Autodesk Inventor part; units mm, degrees
ref_plane "YZ Plane" through (0, 0, 0) normal (1, 0, 0) x (0, 1, 0)
ref_plane "XZ Plane" through (0, 0, 0) normal (0, 1, 0) x (-1, 0, 0)
ref_plane "XY Plane" through (0, 0, 0) normal (0, 0, 1) x (1, 0, 0)
sketch "Sketch1" plane through (0, 0, 0) normal (0, 1, 0) x (-1, 0, 0)
  line L0 (0, 0) -> (0, 29.0928)
  line L1 (0, 29.0928) -> (-0.9185, 29.0928)
  line L2 (-0.9185, 29.0928) -> (-3.25, 24.0928)
  line L3 (-3.25, 24.0928) -> (-2.4, 24.0928)
  line L4 (-2.4, 24.0928) -> (-2.4, 20.2928)
  line L5 (-2.4, 20.2928) -> (-3, 20.2928)
  line L6 (-3, 20.2928) -> (-3, 6)
  line L7 (-3, 6) -> (-1.5, 6)
  line L8 (-1.5, 6) -> (-1.5, 0)
  line L9 (-1.5, 0) -> (0, 0)
  arc A0 (-6.8684, 22.0226) -> (0, 20.2928) centre (0, 34.7935) ccw
  arc A1 (-6.6316, 22.4629) -> (-2.4, 21) centre (0, 34.7935) ccw
  arc A2 (-6.6316, 22.4629) -> (-6.8684, 22.0226) centre (-6.75, 22.2428) ccw
  line L10 (-2.4, 21) -> (0, 21)
  point P0 (0, 10)
  dimension "d0" = 3
  dimension "d1" = 6
  dimension "d3" = 6
  dimension "d4" = 5
  dimension "d5" = 6.5
  dimension "d9" = 8.8
  dimension "d10" = 25
  dimension "d11" = 4.8
  dimension "d15" = 15
  dimension "d17" = 14
  dimension "d18" = 0.5
  dimension "d19" = 1.6
revolve "Revolution1" add sketch "Sketch1" angle 360 about axis through (0, 0, 0) along (0, 0, 1) contours L9 L8 L7 L6 L5 L4 A0 L0 | A0 L4 L10 L0 | L10 L4 L3 L2 L1 L0
extrude "Extrusion1" add sketch "Sketch1" along normal mid plane 5.5 contours A0 L4 L10 L0 | A0 A2 A1 L4
mirror "Mirror1" about plane through (0, 0, 20.2928) normal (-1, 0, 0) of "Extrusion1"
properties part number "WBN-315" material "Acetal Resin, White"
Source: CAD feature listing. Evaluate the final solid. Frame: model axes, mm. A direction names the side the tool comes from. Coordinates: 2 decimals unless noted, no trailing zeros. Order: outer loops, then holes, each group sorted by start corner. A loop starts at its lowest first (then second) coordinate and runs counter-clockwise, first axis right, second up. Notation, with made-up numbers: M 76.5,26 L 132.5,26 A31 cw 132.5,52 Z; hole C -34.5,46.25 d11. An arc over 180 degrees is marked long. Write each question's results on one line, items separated by ' | '. Start each with the question number.
Item 1: First-contact query: pin 1 Ø4 at (x, z) = (-4, 14) entering from -Y; pin 2 Ø1.5 at (x, z) = (3.5, 15.5) entering from +Y; pin 3 Ø8 at (x, z) = (5.5, 14.5) entering from -Y. Flat tips, straight axial feed; report the tip coordinate or a pass-through.
Item 2: Set-up query: faces 1 (the face through (1.3, -1.3, 6)), 2 (the face through (0, 2.75, 20.8)), 3 (the face through (0.01, 2.59, 21)), 4 (the face through (1.29, -2.024, 22.525)), 5 (the face through (4.54, -0.04, 21.55)). Return all of +Z, -Z, +X, -X, +Y, -Y with unobstructed straight access to the full face (end or side cutting, diameter ignored); none if empty.
Item 3: Cut plane A-A (z = 17). Return loops of the section in (x, y).
Item 4: Cut plane B-B (x = -3.75). Return loops of the section in (y, z).
Item 5: Draft query along X for faces 6 (the face through (-1.5, -0.07, 2.96)), 7 (the face through (-4.6, -0.04, 21.57)), 8 (the face through (0, -2.75, 20.8)). Return one class per face: pulls with the +X half, pulls with the -X half, needs draft (parallel to the pull), parting line crosses it, or undercut.
Item 6: Cut plane C-C (x = 6). Return loops of the section in (y, z).
Item 7: Line query: probe 1 along Z at (x, y) = (2.75, 0.5); probe 2 along X at (y, z) = (1.75, 22.25); probe 3 along X at (y, z) = (-0.5, 15.5). Output: solid intervals per line, ascending.
Checked values:
1) pin 1: stops at y = -2.24 | pin 2: stops at y = 1.2 | pin 3: stops at y = -2.6
2) face 1: -Z | face 2: +X, -X, +Y | face 3: +Y | face 4: none | face 5: +Y, -Y
3) outline: C 0,0 d6
4) outline: M -2.75,20.79 L 2.75,20.79 L 2.75,21.3 L -2.75,21.3 Z
5) face 6: parting line crosses it | face 7: undercut | face 8: needs draft
6) outline: M -2.75,21.59 L 2.75,21.59 L 2.75,22.14 L -2.75,22.14 Z
7) probe 1: z = 6 to 20.29, 20.56 to 21.07, 24.09 to 25.07 | probe 2: x = -7 to -6.22, -1.64 to 1.64, 6.22 to 7 | probe 3: x = -2.96 to 2.96
